For this review, take the finished solid that the model builds, in its own axes (mm). A direction names the side the tool comes from. Give positions to 0.01 mm unless a question says otherwise; leave off trailing zeros. Write each loop counter-clockwise with the first axis right and the second up, starting at its lowest first coordinate (ties: lowest second). Pieces come first, ordered by that corner, then holes. Notation, with made-up numbers: M -16,-7 L 17,-7 A26 ccw 17,30 Z; hole C 43.25,55 d5. An arc over 180 degrees is marked long. One line per item, written item: value. Start each with the question number.
Item 1: Consider section C-C, the plane y = 2. Write out the cut boundary in (x, z).
Item 2: Consider section A-A, the plane x = 414. Write out the cut boundary in (y, z) (3 decimals), and give its area (3 significant figures).
Item 3: Mouldability with a two-part tool opening along X and no side actions: class faces 1 (the face through (245, -2.335, -11)), 2 (the face through (521.1, 6, -271)), 3 (the face through (197, -4.335, -539)), 4 (the face through (-78.9, 6, -271)) as released by +X, released by -X, zero draft, split by the parting line, or undercut.
Item 4: Tool access review of faces 5 (the face through (220, -3, 0)), 6 (the face through (519.1, 7, -270)): name each direction out of +Z, -Z, +X, -X, +Y, -Y from which nothing blocks a thin tool from reaching the whole face with its end or side.
Item 5: Consider section B-B, the plane z = -330. Write out the cut boundary in (x, y) (3 decimals), and give its area (3 significant figures).
Item 6: Clearance check with a flat-ended pin moving along its axis: pin 1 Ø9 at (x, y) = (252.5, 4) entering from +Z. State where the tip first meets the part, or that it passes through.
Item 7: To check wall thickness, follow probe 1 along X at (y, z) = (13, -48); probe 2 along X at (y, z) = (-2.5, -362); probe 3 along Z at (x, y) = (376.5, 0). State the ranges of each line that lie inside material, in increasing order.
```python
from build123d import *

# Parameters (mm, degrees)
SKETCH1_W           = 600
SKETCH1_H           = 20
BOSS_EXTRUDE1_DEPTH = 550.1
CUT_EXTRUDE1_DEPTH  = 18
CUT_EXTRUDE2_DEPTH  = 2
SKETCH2_W           = 596
SKETCH2_H           = 18
CUT_EXTRUDE3_DEPTH  = 2


with BuildPart() as part:
    # Sketch1 → Boss-Extrude1 (new body)
    with BuildSketch(Plane.XY):
        with Locations((221.099899989, 5.665003505)):
            Rectangle(SKETCH1_W, SKETCH1_H)
    extrude(amount=-BOSS_EXTRUDE1_DEPTH)

    # 3DSketch1 → Cut-Extrude1 (cut)
    with BuildSketch(Plane(origin=(519.099899989, 15.665003505, -548.1), x_dir=(-0.7372979045405654, 0, 0.6755677611906087), z_dir=(0, 1, 0))):
        Polygon((0, 0), (439.429551106, -402.63838567), (808.357105492, 0), (368.927554386, 402.63838567), align=None)
    extrude(amount=-CUT_EXTRUDE1_DEPTH, mode=Mode.SUBTRACT)

    # 3DSketch2 → Cut-Extrude2 (cut)
    with BuildSketch(Plane(origin=(-58.900100011, -2.334996495, -530.1), x_dir=(0.7392766587492063, 0, 0.6734018279070896), z_dir=(0, 1, 0))):
        Polygon((0, 0), (413.9949289, 377.105023628), (757.497201315, 0), (343.502272415, -377.105023628), align=None)
    extrude(amount=-CUT_EXTRUDE2_DEPTH, mode=Mode.SUBTRACT)

    # Sketch2 → Cut-Extrude3 (cut)
    with BuildSketch(Plane(origin=(0, 0, -2), x_dir=(-1, 0, 0), z_dir=(0, 0, -1))):
        with Locations((-221.099899989, 6.665003505)):
            Rectangle(SKETCH2_W, SKETCH2_H)
    extrude(amount=-CUT_EXTRUDE3_DEPTH, mode=Mode.SUBTRACT)


solid = part.part
```
Model answer:
1. outline: M -78.9,-550.1 L 521.1,-550.1 L 521.1,0 L 519.1,0 L 519.1,-548.1 L -76.9,-548.1 L -76.9,0 L -78.9,0 Z
2. outline: M -4.335,-550.1 L 15.665,-550.1 L 15.665,-548.1 L -2.335,-548.1 L -2.335,-530.1 L -4.335,-530.1 Z; M -4.335,-20 L -2.335,-20 L -2.335,0 L -4.335,0 Z
2. area: 116 mm2
3. face 1: undercut
3. face 2: released by +X
3. face 3: zero draft
3. face 4: released by -X
4. face 5: +Z, +X, -X, +Y, -Y
4. face 6: +Z, +Y
5. outline: M -78.9,-4.335 L -58.9,-4.335 L -58.9,-2.335 L -76.9,-2.335 L -76.9,15.665 L -78.9,15.665 Z; M 501.1,-4.335 L 521.1,-4.335 L 521.1,15.665 L 519.1,15.665 L 519.1,-2.335 L 501.1,-2.335 Z
5. area: 152 mm2
6. pin 1: stops at z = -548.1
7. probe 1: x = -78.9 to -76.9, 519.1 to 521.1
7. probe 2: x = -78.9 to -58.9, 501.1 to 521.1
7. probe 3: z = -550.1 to -548.1
